from build123d import *

# Parameters (mm, degrees)
SKETCH2_R           = 5
BOSS_EXTRUDE1_DEPTH = 10
SKETCH3_R           = 10
SKETCH3_R_2         = 5
BOSS_EXTRUDE2_DEPTH = 76.2
BOSS_EXTRUDE3_START = 86.2
SKETCH2_2_R         = 5
BOSS_EXTRUDE3_DEPTH = 20
SKETCH5_R           = 65
BOSS_EXTRUDE4_DEPTH = 20
SKETCH6_R           = 55
CUT_EXTRUDE1_DEPTH  = 20
SKETCH7_R           = 80
CUT_EXTRUDE2_DEPTH  = 135.370532484
SKETCH8_R           = 7
BOSS_EXTRUDE6_DEPTH = 20
SKETCH9_R           = 7.5
CUT_EXTRUDE3_DEPTH  = 1
CUT_EXTRUDE4_START  = -1
SKETCH10_R          = 7.5
CUT_EXTRUDE4_DEPTH  = 1


with BuildPart() as part:
    # Sketch2 → Boss-Extrude1 (new body)
    with BuildSketch(Plane.XY):
        with BuildLine():
            Line((-19.794866372, 2.857142857), (-9.897433186, 71.428571429))
            ThreePointArc((-9.897433186, 71.428571429), (0, 80), (9.897433186, 71.428571429))
            Line((9.897433186, 71.428571429), (19.794866372, 2.857142857))
            ThreePointArc((19.794866372, 2.857142857), (0, -20), (-19.794866372, 2.857142857))
        make_face()
        with Locations((0, 70)):
            Circle(SKETCH2_R, mode=Mode.SUBTRACT)
        with BuildLine():
            Line((-2.5, 9.682458366), (-2.5, 12))
            Line((-2.5, 12), (2.5, 12))
            Line((2.5, 12), (2.5, 9.682458366))
            ThreePointArc((2.5, 9.682458366), (0, -10), (-2.5, 9.682458366))
        make_face(mode=Mode.SUBTRACT)
    extrude(amount=BOSS_EXTRUDE1_DEPTH)

    # Sketch3 → Boss-Extrude2 (add)
    with BuildSketch(Plane.XY.offset(10)):
        with Locations(Location((0, 70, 0), (0, 0, 171.786789298))):
            Circle(SKETCH3_R)
        with Locations((0, 70)):
            Circle(SKETCH3_R_2, mode=Mode.SUBTRACT)
    extrude(amount=BOSS_EXTRUDE2_DEPTH)

    # Sketch2<2> → Boss-Extrude3 (add)
    with BuildSketch(Plane.XY.offset(BOSS_EXTRUDE3_START)):
        with BuildLine():
            Line((-19.794866372, 2.857142857), (-9.897433186, 71.428571429))
            ThreePointArc((-9.897433186, 71.428571429), (0, 80), (9.897433186, 71.428571429))
            Line((9.897433186, 71.428571429), (19.794866372, 2.857142857))
            ThreePointArc((19.794866372, 2.857142857), (0, -20), (-19.794866372, 2.857142857))
        make_face()
        with Locations((0, 70)):
            Circle(SKETCH2_2_R, mode=Mode.SUBTRACT)
        with BuildLine():
            Line((-2.5, 9.682458366), (-2.5, 12))
            Line((-2.5, 12), (2.5, 12))
            Line((2.5, 12), (2.5, 9.682458366))
            ThreePointArc((2.5, 9.682458366), (0, -10), (-2.5, 9.682458366))
        make_face(mode=Mode.SUBTRACT)
    extrude(amount=BOSS_EXTRUDE3_DEPTH)

    # Sketch5 → Boss-Extrude4 (add)
    with BuildSketch(Plane.XY.offset(106.2)):
        Circle(SKETCH5_R)
    extrude(amount=-BOSS_EXTRUDE4_DEPTH)

    # Sketch6 → Cut-Extrude1 (cut)
    with BuildSketch(Plane.XY.offset(106.2)):
        Circle(SKETCH6_R)
    extrude(amount=-CUT_EXTRUDE1_DEPTH, mode=Mode.SUBTRACT)

    # Sketch7 → Cut-Extrude2 (cut, through all)
    with BuildSketch(Plane(origin=(0, 0, 86.2), x_dir=(-1, 0, 0), z_dir=(0, 0, -1))):
        Circle(SKETCH7_R)
    extrude(amount=CUT_EXTRUDE2_DEPTH, mode=Mode.SUBTRACT)

    # Sketch8 → Boss-Extrude6 (add)
    with BuildSketch(Plane.XY.offset(106.2)):
        with BuildLine():
            Line((-17.860571099, 109), (-58.046856073, 29.25))
            ThreePointArc((-58.046856073, 29.25), (-38.646753366, 52.263069698), (-10.959640032, 64.06938653))
            Line((-10.959640032, 64.06938653), (-9.897433186, 71.428571429))
            ThreePointArc((-9.897433186, 71.428571429), (0, 80), (9.897433186, 71.428571429))
            Line((9.897433186, 71.428571429), (10.959640032, 64.06938653))
            ThreePointArc((10.959640032, 64.06938653), (38.646753366, 52.263069698), (58.046856073, 29.25))
            Line((58.046856073, 29.25), (17.860571099, 109))
            ThreePointArc((17.860571099, 109), (0, 120), (-17.860571099, 109))
        make_face()
        with Locations((0, 100)):
            Circle(SKETCH8_R, mode=Mode.SUBTRACT)
    extrude(amount=-BOSS_EXTRUDE6_DEPTH)

    # Sketch9 → Cut-Extrude3 (cut)
    with BuildSketch(Plane.XY.offset(106.2)):
        with Locations((0, 100)):
            Circle(SKETCH9_R)
    extrude(amount=-CUT_EXTRUDE3_DEPTH, mode=Mode.SUBTRACT)

    # Sketch10 → Cut-Extrude4 (cut)
    with BuildSketch(Plane(origin=(0, 0, 86.2), x_dir=(-1, 0, 0), z_dir=(0, 0, -1)).offset(CUT_EXTRUDE4_START)):
        with Locations(Location((0, 100, 0), (0, 0, 180))):
            Circle(SKETCH10_R)
    extrude(amount=CUT_EXTRUDE4_DEPTH, mode=Mode.SUBTRACT)


solid = part.part
Read the model definition and answer for the solid it produces. Units are mm, in the model's axes. A direction names the side the tool comes from. Give positions to 0.01 mm unless a question says otherwise; leave off trailing zeros. Loops run counter-clockwise (first coordinate to the right, second up) from the corner with the lowest first, then second, coordinate; pieces in that order, holes last. Notation, with made-up numbers: (68.5, -40) - (121.5, -40) arc R19 ccw to (121.5, -18) - close; hole circle Ø8 at (66.5, 17). An arc over 180 degrees is marked (long way). Answer as CSV lines item,"result". Start each with the question number.
1) Find section D-D (x = 30). Write down the section's boundary in (y, z).
2) Each of these flat-tipped pins is pushed along its axis until it touches: pin 1 Ø8 at (x, z) = (49.5, 102.5) entering from +Y; pin 2 Ø2 at (x, z) = (-21, 95.5) entering from -Y; pin 3 Ø1.5 at (y, z) = (2, 95.5) entering from -X; pin 4 Ø8.5 at (x, y) = (0, 100) entering from -Z. Where does it stop, or does it pass through?
3) Find section C-C (y = -5.5). Write down the section's boundary in (x, z).
4) Find section A-A (x = 0). Write down the section's boundary in (y, z).
5) Straight lines are drawn through the part: L1, parallel to X at y = -26.5, z = 96; L2, parallel to X at y = 70, z = 100.5; L3, parallel to Y at x = 39, z = 94. For each, find the intervals that lie inside material, in ascending order. Write a range as from..to.
6) Determine the mould class of faces 4 (the face through (-0.3, 55.3, 106.2)), 5 (the face through (0, 120, 96)), 6 (the face through (-0.91, 106.94, 96.33)) for opening direction X: released by +X, released by -X, zero draft, split by the parting line, or undercut.
7) Find section B-B (z = 100.25). Write down the section's boundary in (x, y), then the cut area to 3 significant figures.
8) Which of the six approach directions +Z, -Z, +X, -X, +Y, -Y give full straight-line access (tool end or side, diameter ignored) to faces 1 (the face through (-2, 107, 87.2)), 2 (the face through (-11.923, -53.692, 96.34)), 3 (the face through (-1.63, 92.68, 105.71))?
Findings below:
1,outline,"(-57.66, 86.2) - (-46.1, 86.2) - (-46.1, 106.2) - (-57.66, 106.2) - close; (46.1, 86.2) - (84.91, 86.2) - (84.91, 106.2) - (46.1, 106.2) - close"
2,pin 1,"y = 54.15"
2,pin 2,"y = -61.85"
2,pin 3,"x = -64.99"
2,pin 4,"through"
3,outline,"(-64.77, 86.2) - (-54.72, 86.2) - (-54.72, 106.2) - (-64.77, 106.2) - close; (54.72, 86.2) - (64.77, 86.2) - (64.77, 106.2) - (54.72, 106.2) - close"
4,outline,"(-65, 86.2) - (-55, 86.2) - (-55, 106.2) - (-65, 106.2) - close; (55, 86.2) - (65, 86.2) - (65, 106.2) - (55, 106.2) - close; (75, 86.2) - (92.5, 86.2) - (92.5, 87.2) - (93, 87.2) - (93, 105.2) - (92.5, 105.2) - (92.5, 106.2) - (75, 106.2) - close; (107, 87.2) - (107.5, 87.2) - (107.5, 86.2) - (120, 86.2) - (120, 106.2) - (107.5, 106.2) - (107.5, 105.2) - (107, 105.2) - close"
5,L1,"-59.35..-48.19, 48.19..59.35"
5,L2,"-37.51..-5, 5..37.51"
5,L3,"-52..-38.78, 38.78..67.05"
6,face 4,"zero draft"
6,face 5,"split by the parting line"
6,face 6,"undercut"
7,outline,"(-58.05, 29.25) arc R65 ccw (long way) to (58.05, 29.25) - (17.86, 109) arc R20 ccw to (-17.86, 109) - close; hole circle Ø110 at (0, 0); hole circle Ø14 at (0, 100); hole circle Ø10 at (0, 70)"
7,area,"6,910 mm^2"
8,face 1,"-Z"
8,face 2,"+Z, -Z"
8,face 3,"+Z"
